Autodesk Inventor part; units mm, degrees
ref_plane "XZ Plane" through (0, 0, 0) normal (0, 1, 0) x (-1, 0, 0)
ref_plane "XY Plane" through (0, 0, 0) normal (0, 0, 1) x (1, 0, 0)
sketch "Schizzo1" plane through (0, 0, 0) normal (0, 1, 0) x (-1, 0, 0)
  circle A0 centre (1.635, 2.2831) radius 4
  dimension "d2" = 8
extrude "Estrusione1" add sketch "Schizzo1" along normal blind 10
thread "Filettatura1"
sketch "Schizzo2" plane through (-1.635, 0, 2.2831) normal (0, -1, 0) x (1, 0, 0)
  point P0 (1.635, -2.2831)
  point P1 (0, 0)
hole "Foro1" at (-1.635, 0, 2.2831) direction (0, 1, 0) diameter 4 end through all
thread "Filettatura2"
chamfer "Smusso1" distance 0.8 distance2 2 2 edges at (2.365, 0, 2.2831) (2.365, 10, 2.2831) measured on face at (-5.5832, 6.6667, 1.6415)
ref_plane "Piano di lavoro1" through (2.365, 0, 2.2831) normal (1, 0, 0) x (0, 1, 0)
sketch "Schizzo3" plane through (2.365, 0, 2.2831) normal (1, 0, 0) x (0, 1, 0)
  line L0 (10, 2) -> (10, -2)
  line L1 (0, -2) -> (0, 2)
  line L2 (9.2, -4) -> (9.2, 4)
  line L3 (0.8, 4) -> (0.8, -4)
  line L4 (10, -0.5) -> (9.2, -0.5)
  line L5 (9.2, -0.5) -> (9.2, 0.5)
  line L6 (9.2, 0.5) -> (10, 0.5)
  line L7 (10, 0.5) -> (10, -0.5)
  line L8 (0, 0) -> (10, 0)
  line L9 (0.8, -0.5) -> (0, -0.5)
  line L10 (0, -0.5) -> (0, 0.5)
  line L11 (0, 0.5) -> (0.8, 0.5)
  line L12 (0.8, 0.5) -> (0.8, -0.5)
  point P0 (0, -2.2831)
  point P1 (0.8, 0.5)
  point P2 (0, -0.5)
  dimension "d19" = 1
extrude "Estrusione2" cut sketch "Schizzo3" along normal through all both and the other way through all
properties part number "M8x1.25-M4x0.7 Thread Reductor"
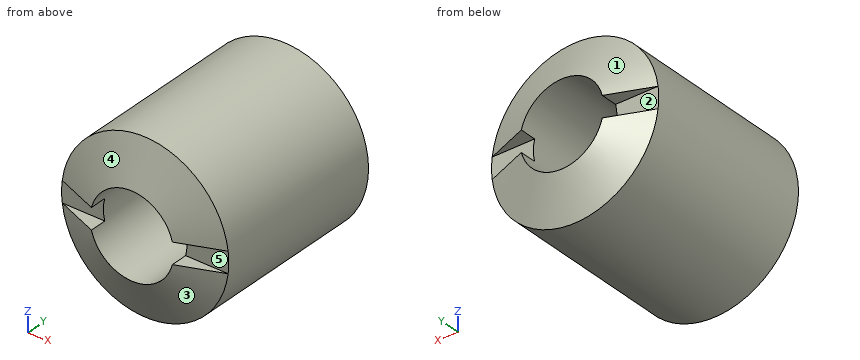
Geometry check sheet. Reference: the model listing, model coordinates, mm. Face numbers are marked on the shaded views. A direction names the side the tool comes from. Give positions to 0.01 mm unless a question says otherwise; leave off trailing zeros. Order: outer loops, then holes, each group sorted by start corner. A loop starts at its lowest first (then second) coordinate and runs counter-clockwise, first axis right, second up.
1. Section check C-C, the plane y = 2.25. Enter the section's corners in (x, z) (3 decimals).
2. Thickness scan on L1, parallel to Y at x = 1.5, z = 2.25; L2, parallel to X at y = 2, z = 3; L3, parallel to Z at x = -2.25, y = 1.5. Record the ranges inside material, lowest first.
3. Section check A-A, the plane z = 2. Enter the section's corners in (x, y).
4. Gauge pin test, flat ends, axial feed: pin 1 Ø0.9 at (x, y) = (1, 9.5) entering from +Z; pin 2 Ø0.9 at (x, y) = (-4.5, 9.5) entering from -Z; pin 3 Ø3 at (x, y) = (0, 4) entering from +Z. Record the tip position at first contact, or that the pin passes through.
5. Access from +Z, -Z, +X, -X, +Y, -Y to the whole of each face (thin tool, end or side, straight path). Record for the marked faces 1 and 2.
6. Release check for a two-part mould opening along Z. For the marked faces 3, 4 and 5 record: pulls with the +Z half, pulls with the -Z half, needs draft (parallel to the pull), parting line crosses it, or undercut.
Values follow:
1. outline: circle Ø8 at (-1.635, 2.283); hole circle Ø4 at (-1.635, 2.283)
2. L1: y = 0.8 to 9.2
2. L2: x = -5.57 to -3.5, 0.23 to 2.3
2. L3: z = -1.67 to 0.38, 4.19 to 6.24
3. outline: (-5.62, 0.8) - (-3.61, 0.8) - (-3.61, 9.2) - (-5.62, 9.2) - close; (0.34, 0.8) - (2.35, 0.8) - (2.35, 9.2) - (0.34, 9.2) - close
4. pin 1: stops at z = 5.56
4. pin 2: stops at z = -0.82
4. pin 3: stops at z = 6.28
5. face 1: +Z, +Y
5. face 2: +X, -X, +Y
6. face 3: pulls with the -Z half
6. face 4: pulls with the +Z half
6. face 5: undercut
